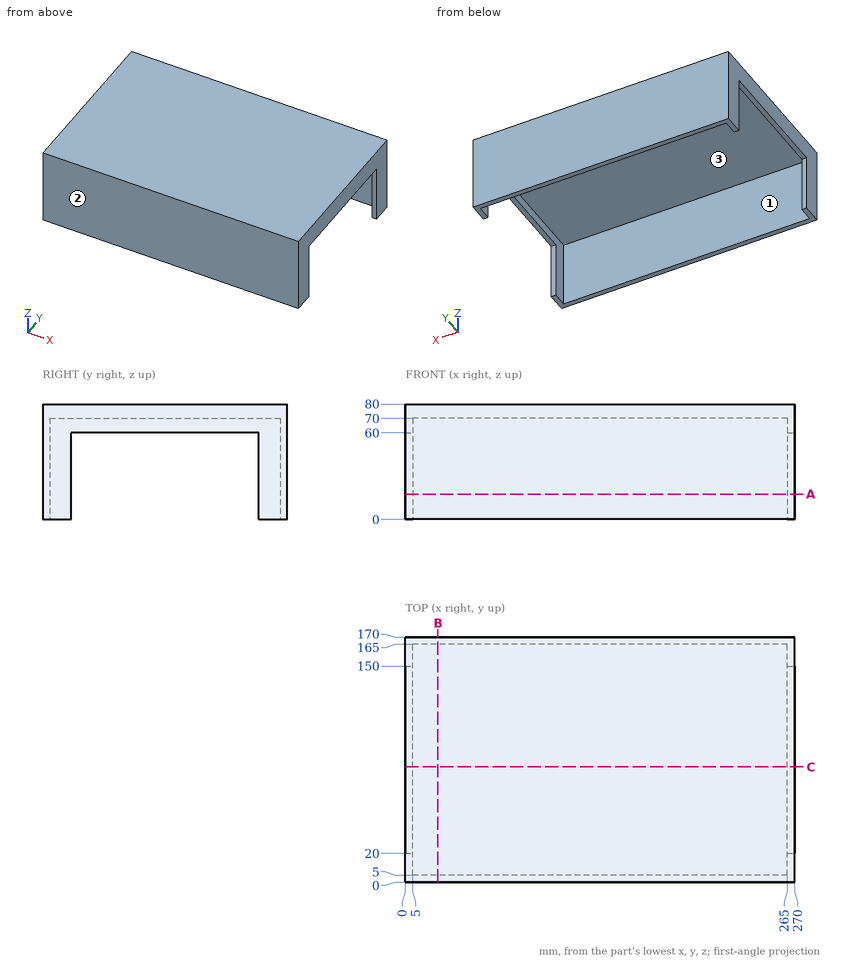
Part print with two shaded views. Sizes in mm from the minimum x, y, z corner. Round coordinates to 2 decimals unless told otherwise and drop trailing zeros. Order: outer loops, then holes, each group sorted by start corner. A loop starts at its lowest first (then second) coordinate and runs counter-clockwise, first axis right, second up. Notation, with made-up numbers: M -38.5,20.5 L -2.5,20.5 A26 ccw -2.5,37.5 Z; hole C 13.5,-30.5 d5. An arc over 180 degrees is marked long. Use CSV: the item, a comma, the result in double quotes.
Item 1: Saw through at A-A (z = 17.5). List the corners of the cut face in (x, y).
Worked answers:
outline,"M 0,0 L 270,0 L 270,20 L 265,20 L 265,5 L 5,5 L 5,20 L 0,20 Z; M 0,150 L 5,150 L 5,165 L 265,165 L 265,150 L 270,150 L 270,170 L 0,170 Z"
Item 2: Pin check, flat tips, straight feed: pin 1 (2.5 mm diameter, centred on x = 2, z = 29.5, fed in from -Y); pin 2 (2.5 mm diameter, centred on x = 267, y = 78, fed in from -Z); pin 3 (1.5 mm diameter, centred on x = 232, y = 73, fed in from -Z). Stop position of each tip, or through.
Worked answers:
pin 1,"y = 0"
pin 2,"z = 60"
pin 3,"z = 70"
Item 3: Probe probe 1 along Y at (x, z) = (219.5, 21); probe 2 along Z at (x, y) = (246.5, 57.5). List the from-to ranges inside material, lowest first.
Worked answers:
probe 1,"0 to 5, 165 to 170"
probe 2,"70 to 80"
Item 4: Saw through at B-B (x = 22.5). List the corners of the cut face in (y, z).
Worked answers:
outline,"M 0,0 L 5,0 L 5,70 L 165,70 L 165,0 L 170,0 L 170,80 L 0,80 Z"
Item 5: Saw through at C-C (y = 80). List the corners of the cut face in (x, z).
Worked answers:
outline,"M 0,60 L 5,60 L 5,70 L 265,70 L 265,60 L 270,60 L 270,80 L 0,80 Z"
Item 6: Pull direction X, two halves, no side cores. Call the marked faces 1, 2 and 3: released by +X, released by -X, zero draft, split by the parting line, or undercut.
Worked answers:
face 1,"undercut"
face 2,"zero draft"
face 3,"undercut"
